Design review of the part built by this model. Coordinates are the model's own, in mm. A direction names the side the tool comes from. Coordinates: 2 decimals unless noted, no trailing zeros. Write each loop counter-clockwise with the first axis right and the second up, starting at its lowest first coordinate (ties: lowest second). Pieces come first, ordered by that corner, then holes. Notation, with made-up numbers: M 64.5,-36.5 L 76.5,-36.5 A24 ccw 76.5,-23.5 Z; hole C 2.5,-38.75 d8. An arc over 180 degrees is marked long. One line per question, with ' | ' between items.
from build123d import *

# Parameters (mm, degrees)
SALIENTE_EXTRUIR2_DEPTH = 22
SALIENTE_EXTRUIR3_DEPTH = 2
CORTAR_EXTRUIR1_DEPTH   = 2
CHAFL_N1_SIZE           = 3
REDONDEO2_R             = 3
CROQUIS4_W              = 22.9
CROQUIS4_H              = 10.4
CORTAR_EXTRUIR2_DEPTH   = 10
CROQUIS5_W              = 14.5
CROQUIS5_H              = 8.9
CORTAR_EXTRUIR3_DEPTH   = 10


# Some blends are built 0.0001 mm under size
with BuildPart() as part:
    # Croquis1 → Saliente-Extruir2 (new body)
    with BuildSketch(Plane(origin=(0, 0, 0), x_dir=(1, 0, 0), z_dir=(0, 1, 0))):
        with BuildLine():
            Line((-52.8, 29.5), (52.8, 29.5))
            ThreePointArc((52.8, 29.5), (57.891168825, 27.391168825), (60, 22.3))
            Line((60, 22.3), (60, -22.3))
            ThreePointArc((60, -22.3), (57.891168825, -27.391168825), (52.8, -29.5))
            Line((52.8, -29.5), (-52.8, -29.5))
            ThreePointArc((-52.8, -29.5), (-57.891168825, -27.391168825), (-60, -22.3))
            Line((-60, -22.3), (-60, 22.3))
            ThreePointArc((-60, 22.3), (-57.891168825, 27.391168825), (-52.8, 29.5))
        make_face()
        with BuildLine():
            Line((-52.225351705, 26.5), (52.225351705, 26.5))
            ThreePointArc((52.225351705, 26.5), (55.601537892, 25.101537892), (57, 21.725351705))
            Line((57, 21.725351705), (57, -21.725351705))
            ThreePointArc((57, -21.725351705), (55.601537892, -25.101537892), (52.225351705, -26.5))
            Line((52.225351705, -26.5), (-52.225351705, -26.5))
            ThreePointArc((-52.225351705, -26.5), (-55.601537892, -25.101537892), (-57, -21.725351705))
            Line((-57, -21.725351705), (-57, 21.725351705))
            ThreePointArc((-57, 21.725351705), (-55.601537892, 25.101537892), (-52.225351705, 26.5))
        make_face(mode=Mode.SUBTRACT)
    extrude(amount=SALIENTE_EXTRUIR2_DEPTH)

    # Croquis2 → Saliente-Extruir3 (add)
    with BuildSketch(Plane.XZ):
        with BuildLine():
            Line((-60, 22.3), (-60, -22.3))
            ThreePointArc((-60, -22.3), (-57.891168825, -27.391168825), (-52.8, -29.5))
            Line((-52.8, -29.5), (52.8, -29.5))
            ThreePointArc((52.8, -29.5), (57.891168825, -27.391168825), (60, -22.3))
            Line((60, -22.3), (60, 22.3))
            ThreePointArc((60, 22.3), (57.891168825, 27.391168825), (52.8, 29.5))
            Line((52.8, 29.5), (-52.8, 29.5))
            ThreePointArc((-52.8, 29.5), (-57.891168825, 27.391168825), (-60, 22.3))
        make_face()
    extrude(amount=-SALIENTE_EXTRUIR3_DEPTH)

    # Croquis3 → Cortar-Extruir1 (cut)
    with BuildSketch(Plane(origin=(0, 2, 0), x_dir=(1, 0, 0), z_dir=(0, 1, 0))):
        with BuildLine():
            Line((-46, 20), (46, 20))
            ThreePointArc((46, 20), (48.828427125, 18.828427125), (50, 16))
            Line((50, 16), (50, -16))
            ThreePointArc((50, -16), (48.828427125, -18.828427125), (46, -20))
            Line((46, -20), (-46, -20))
            ThreePointArc((-46, -20), (-48.828427125, -18.828427125), (-50, -16))
            Line((-50, -16), (-50, 16))
            ThreePointArc((-50, 16), (-48.828427125, 18.828427125), (-46, 20))
        make_face()
    extrude(amount=-CORTAR_EXTRUIR1_DEPTH, mode=Mode.SUBTRACT)

    # Chaflán1
    # the kernel refuses this chamfer: 3 mm, written as the material it takes off along each edge
    with BuildSketch(Plane(origin=(-50, 0, 16), x_dir=(-0.9996219169112968, -0.02749587661058636, 0), z_dir=(0, 0, -1)), Plane(origin=(50, 0, -16), x_dir=(0.9996219169112968, -0.02749587661058636, 0), z_dir=(0, 0, 1))) as chafl_n1_piece_1:
        Polygon((CHAFL_N1_SIZE * 0.999621916911, CHAFL_N1_SIZE * 0.0274958766106), (-CHAFL_N1_SIZE * 0.0274958766106, CHAFL_N1_SIZE * 0.999621916911), (0, 0), align=None)
    extrude(amount=32, mode=Mode.SUBTRACT)
    with BuildSketch(Plane(origin=(-46, 0, 16), x_dir=(0, 0, 1), z_dir=(1, 0, 0))) as chafl_n1_piece_2:
        Polygon((4 + CHAFL_N1_SIZE, 0), (4, -CHAFL_N1_SIZE), (4, 0), align=None)
    revolve(axis=Axis((-46, 0, 16), (0, -1, 0)), revolution_arc=90, mode=Mode.SUBTRACT)
    with BuildSketch(Plane(origin=(-46, 0, -16), x_dir=(-1, 0, 0), z_dir=(0, 0, 1))) as chafl_n1_piece_3:
        Polygon((4 + CHAFL_N1_SIZE, 0), (4, -CHAFL_N1_SIZE), (4, 0), align=None)
    revolve(axis=Axis((-46, 0, -16), (0, -1, 0)), revolution_arc=90, mode=Mode.SUBTRACT)
    with BuildSketch(Plane(origin=(46, 0, 20), x_dir=(0, -0.02749587661058636, 0.9996219169112968), z_dir=(-1, 0, 0)), Plane(origin=(-46, 0, -20), x_dir=(0, -0.02749587661058636, -0.9996219169112968), z_dir=(1, 0, 0))) as chafl_n1_piece_4:
        Polygon((CHAFL_N1_SIZE * 0.999621916911, CHAFL_N1_SIZE * 0.0274958766106), (-CHAFL_N1_SIZE * 0.0274958766106, CHAFL_N1_SIZE * 0.999621916911), (0, 0), align=None)
    extrude(amount=92, mode=Mode.SUBTRACT)
    with BuildSketch(Plane(origin=(46, 0, 16), x_dir=(1, 0, 0), z_dir=(0, 0, -1))) as chafl_n1_piece_5:
        Polygon((4 + CHAFL_N1_SIZE, 0), (4, -CHAFL_N1_SIZE), (4, 0), align=None)
    revolve(axis=Axis((46, 0, 16), (0, -1, 0)), revolution_arc=90, mode=Mode.SUBTRACT)
    with BuildSketch(Plane(origin=(46, 0, -16), x_dir=(0, 0, -1), z_dir=(-1, 0, 0))) as chafl_n1_piece_6:
        Polygon((4 + CHAFL_N1_SIZE, 0), (4, -CHAFL_N1_SIZE), (4, 0), align=None)
    revolve(axis=Axis((46, 0, -16), (0, -1, 0)), revolution_arc=90, mode=Mode.SUBTRACT)

    # Redondeo2
    redondeo2_edges = [part.edges().sort_by_distance(p)[0] for p in [
        (57.891168825, 22, 27.391168825),
        (60, 22, 0),
        (57.891168825, 22, -27.391168825),
        (0, 22, -29.5),
        (-57.891168825, 22, -27.391168825),
        (-60, 22, 0),
        (-57.891168825, 22, 27.391168825),
        (0, 22, 29.5),
    ]]
    fillet(redondeo2_edges, radius=REDONDEO2_R - 0.0001)  # a hair under: the kernel refuses the full size

    # Croquis4 → Cortar-Extruir2 (cut)
    with BuildSketch(Plane(origin=(60, 0, 0), x_dir=(0, 0, -1), z_dir=(1, 0, 0))):
        with Locations((0, 13.8)):
            Rectangle(CROQUIS4_W, CROQUIS4_H)
    extrude(amount=-CORTAR_EXTRUIR2_DEPTH, mode=Mode.SUBTRACT)

    # Croquis5 → Cortar-Extruir3 (cut)
    with BuildSketch(Plane(origin=(0, 0, -29.5), x_dir=(-1, 0, 0), z_dir=(0, 0, -1))):
        with Locations((36.55, 14.55)):
            Rectangle(CROQUIS5_W, CROQUIS5_H)
    extrude(amount=-CORTAR_EXTRUIR3_DEPTH, mode=Mode.SUBTRACT)


solid = part.part
1. To check wall thickness, follow line 1 along Z through (x, y) = (-33, 6.25); line 2 along X through (y, z) = (7.25, -12.5); line 3 along X through (y, z) = (9.5, 5). State the ranges of each line that lie inside material, in increasing order. Write a range as [from, to].
Answer sheet:
line 1: [-29.5, -26.5], [26.5, 29.5] | line 2: [-60, -57], [57, 60] | line 3: [-60, -57]
2. Draft analysis for pull direction X (two halves, no side actions). For faces 6 (the face through (0, 0, -24)), 7 (the face through (55.56, 11.86, -25.14)), 8 (the face through (-60, 9, 0)), 9 (the face through (-50.12, 1.236, -20.031)), state which applies: pulls with the +X half, pulls with the -X half, needs draft (parallel to the pull), parting line crosses it, or undercut.
Answer sheet:
face 6: needs draft | face 7: undercut | face 8: pulls with the -X half | face 9: undercut
3. Tool access review of faces 1 (the face through (-36, 19, -28)), 2 (the face through (50.031, 1.236, -20.12)), 3 (the face through (-57, 12, 0)), 4 (the face through (59, 8.6, 0)), 5 (the face through (57.95, 9.37, 27.33)): name each direction out of +Z, -Z, +X, -X, +Y, -Y from which nothing blocks a thin tool from reaching the whole face with its end or side.
Answer sheet:
face 1: -Z | face 2: -Y | face 3: +Y | face 4: +X | face 5: +Z, +X, +Y, -Y
4. Insertion check: pin 1 Ø1.5 at (x, y) = (59, 13.5) entering from -Z; pin 2 Ø1.5 at (x, y) = (58.5, 13.5) entering from +Z; pin 3 Ø1.5 at (x, z) = (10, 19) entering from -Y; pin 4 Ø0.9 at (x, z) = (-34, -27.5) entering from +Y. Each pin has a flat end and moves straight along its axis. Give the tip position at first contact, or say it passes through.
Answer sheet:
pin 1: z = -27.01 | pin 2: z = 27.53 | pin 3: through | pin 4: y = 21.95
5. Take a section at D-D (y = 11.25). Write out the cut boundary in (x, z), then the cut area to 3 significant figures.
Answer sheet:
outline: M -60,-22.3 A7.2 ccw -52.8,-29.5 L -43.8,-29.5 L -43.8,-26.5 L -52.23,-26.5 A4.77 cw -57,-21.73 L -57,21.73 A4.77 cw -52.23,26.5 L 52.23,26.5 A4.77 cw 57,21.73 L 57,11.45 L 60,11.45 L 60,22.3 A7.2 ccw 52.8,29.5 L -52.8,29.5 A7.2 ccw -60,22.3 Z; M -29.3,-29.5 L 52.8,-29.5 A7.2 ccw 60,-22.3 L 60,-11.45 L 57,-11.45 L 57,-21.73 A4.77 cw 52.23,-26.5 L -29.3,-26.5 Z | area: 901 mm^2
6. Take a section at A-A (z = 2). Count the separate pieces of the cut face and the enclosed holes in it, then the cut area to 3 significant figures.
Answer sheet:
separate pieces: 3 | enclosed holes: 0 | area: 117 mm^2
7. Take a section at B-B (y = 4.5). Write out the cut boundary in (x, z), then the cut area to 3 significant figures.
Answer sheet:
outline: M -60,-22.3 A7.2 ccw -52.8,-29.5 L 52.8,-29.5 A7.2 ccw 60,-22.3 L 60,22.3 A7.2 ccw 52.8,29.5 L -52.8,29.5 A7.2 ccw -60,22.3 Z; hole M -57,-21.73 A4.77 ccw -52.23,-26.5 L 52.23,-26.5 A4.77 ccw 57,-21.73 L 57,21.73 A4.77 ccw 52.23,26.5 L -52.23,26.5 A4.77 ccw -57,21.73 Z | area: 1,010 mm^2
